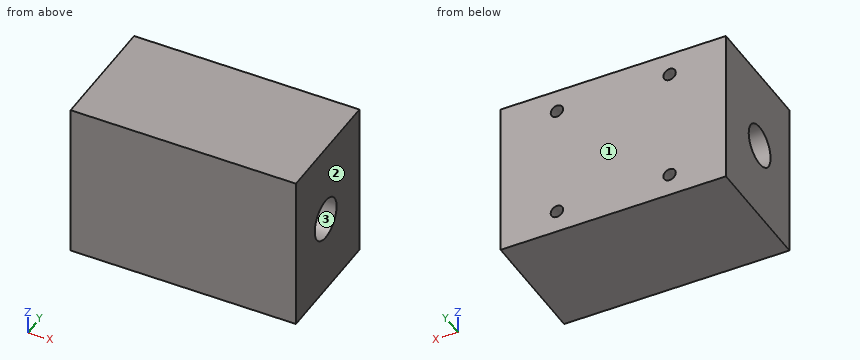
```python
from build123d import *

# Parameters (mm, degrees)
SKETCH1_W                 = 60
SKETCH1_H                 = 42
BOSS_EXTRUDE1_DEPTH       = 32
M4X0_7_TAPPED_HOLE1_D     = 3.3
M4X0_7_TAPPED_HOLE1_DEPTH = 15
M4X0_7_TAPPED_HOLE1_TIP   = 0.991420021
SKETCH4_R                 = 5.5
CUT_EXTRUDE1_DEPTH        = 72.168813395


with BuildPart() as part:
    # Sketch1 → Boss-Extrude1 (new body)
    with BuildSketch(Plane(origin=(0, 0, 0), x_dir=(1, 0, 0), z_dir=(0, 1, 0))):
        Rectangle(SKETCH1_W, SKETCH1_H)
    extrude(amount=BOSS_EXTRUDE1_DEPTH)

    # M4x0.7 Tapped Hole1
    with Locations(Plane(origin=(0, 32, 0), x_dir=(1, 0, 0), z_dir=(0, 1, 0))):
        with Locations((15, 15), (-15, 15), (-15, -15), (15, -15)):
            Hole(M4X0_7_TAPPED_HOLE1_D / 2, depth=M4X0_7_TAPPED_HOLE1_DEPTH)
            with Locations((0, 0, -(M4X0_7_TAPPED_HOLE1_DEPTH + M4X0_7_TAPPED_HOLE1_TIP / 2))):  # 118° drill point
                Cone(0, M4X0_7_TAPPED_HOLE1_D / 2, M4X0_7_TAPPED_HOLE1_TIP, mode=Mode.SUBTRACT)

    # Sketch4 → Cut-Extrude1 (cut, through all)
    with BuildSketch(Plane(origin=(30, 0, 0), x_dir=(0, 0, -1), z_dir=(1, 0, 0))):
        with Locations((0, 15)):
            Circle(SKETCH4_R)
    extrude(amount=-CUT_EXTRUDE1_DEPTH, mode=Mode.SUBTRACT)


solid = part.part
```
Model file for the job. Use its own axes, mm. Face numbers are marked on the shaded views. Coordinates: 2 decimals unless noted, no trailing zeros. Loops run counter-clockwise (first coordinate to the right, second up) from the corner with the lowest first, then second, coordinate; pieces in that order, holes last. Notation, with made-up numbers: (37.25, -32) - (75.25, -32) arc R31 ccw to (75.25, -8) - close; hole circle Ø10 at (0, -23.75). An arc over 180 degrees is marked (long way). Write item = value, one per line. Start each with the question number.
Item 1: Pull direction Y, two halves, no side cores. Call the marked faces 1, 2 and 3: +Y half, -Y half, draft (parallel to the pull), parting line (faces both ways), or undercut.
Item 2: Saw through at B-B, the plane z = 0. List the corners of the cut face in (x, y), then the cut area to 3 significant figures.
Item 3: Saw through at A-A, the plane y = 15. List the corners of the cut face in (x, z), then the cut area to 3 significant figures.
Item 4: Wall check: probe 1 along X at (y, z) = (25, 15); probe 2 along Z at (x, y) = (15, 25); probe 3 along Y at (x, z) = (2.5, 0). Give the ranges that are in metal, low to high. Write a range as [from, to].
Item 5: Saw through at D-D, the plane x = -19.5. List the corners of the cut face in (y, z).
Item 6: Saw through at C-C, the plane y = 19.5. List the corners of the cut face in (x, z), then the cut area to 3 significant figures.
Answers:
q1.face_1 = +Y half
q1.face_2 = draft
q1.face_3 = undercut
q2.outline = (-30, 0) - (30, 0) - (30, 9.5) - (-30, 9.5) - close; (-30, 20.5) - (30, 20.5) - (30, 32) - (-30, 32) - close
q2.area = 1,260 mm2
q3.outline = (-30, -21) - (30, -21) - (30, -5.5) - (-30, -5.5) - close; (-30, 5.5) - (30, 5.5) - (30, 21) - (-30, 21) - close
q3.area = 1,860 mm2
q4.probe_1 = [-30, -16.65], [-13.35, 13.35], [16.65, 30]
q4.probe_2 = [-21, -16.65], [-13.35, 13.35], [16.65, 21]
q4.probe_3 = [0, 9.5], [20.5, 32]
q5.outline = (0, -21) - (32, -21) - (32, 21) - (0, 21) - close; hole circle Ø11 at (15, 0)
q6.outline = (-30, -21) - (30, -21) - (30, -3.16) - (-30, -3.16) - close; (-30, 3.16) - (30, 3.16) - (30, 21) - (-30, 21) - close; hole circle Ø3.3 at (-15, -15); hole circle Ø3.3 at (-15, 15); hole circle Ø3.3 at (15, -15); hole circle Ø3.3 at (15, 15)
q6.area = 2,110 mm2
